Could you check a few things on this drawing? It's one solid part, dimensions in mm from its lowest x, y, z. A direction names the side the tool comes from. Give positions to 0.01 mm unless a question says otherwise; leave off trailing zeros. Loops run counter-clockwise (first coordinate to the right, second up) from the corner with the lowest first, then second, coordinate; pieces in that order, holes last.
Q1. I need wall thicknesses on probe 1 along Z at (x, y) = (25, 24); probe 2 along Z at (x, y) = (26.5, 2); probe 3 along Y at (x, z) = (19, 37.5). Which ranges of each line are inside material? Lowest first, please.
Q2. I'm going to push flat-ended pins straight in: P1, Ø6, axis at x = 31.5, y = 6.5, coming from the -Z side; P2, Ø1.3, axis at y = 17.5, z = 48.5, coming from the +X side; P3, Ø5, axis at x = 7, z = 20.5, coming from the +Y side; P4, Ø1.5, axis at x = 19.5, z = 24.5, coming from the +Y side. Where does each tip first touch, or does it pass through?
Q3. Suppose I cut it at B-B (x = 18.5). List the corners of the cut face in (y, z) for me, and give its area (3 significant figures).
Q4. Suppose I cut it at D-D (y = 23). List the corners of the cut face in (x, z) for me, and give its area (3 significant figures).
Q5. Suppose I cut it at A-A (y = 18.5). List the corners of the cut face in (x, z) for me.
Q6. For the marked faces 1 and 2, which set-ups out of +Z, -Z, +X, -X, +Y, -Y let a thin tool reach every point of the face, with its end or its side?
Q7. Suppose I cut it at C-C (z = 36). List the corners of the cut face in (x, y) for me, and give its area (3 significant figures).
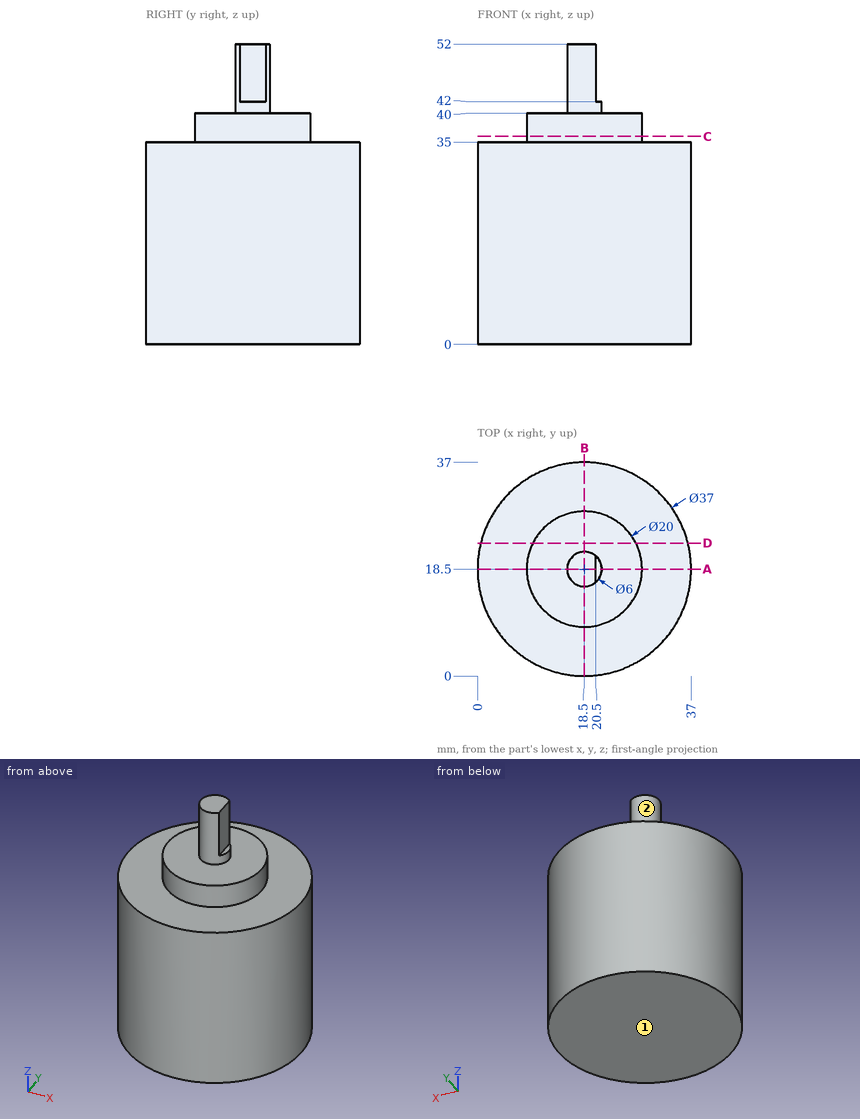
Solutions:
1. probe 1: z = 0 to 40
1. probe 2: z = 0 to 35
1. probe 3: y = 8.51 to 28.49
2. P1: stops at z = 0
2. P2: stops at x = 20.5
2. P3: stops at y = 34.66
2. P4: stops at y = 37
3. outline: (0, 0) - (37, 0) - (37, 35) - (28.5, 35) - (28.5, 40) - (21.5, 40) - (21.5, 52) - (15.5, 52) - (15.5, 40) - (8.5, 40) - (8.5, 35) - (0, 35) - close
3. area: 1,470 mm2
4. outline: (0.56, 0) - (36.44, 0) - (36.44, 35) - (27.43, 35) - (27.43, 40) - (9.57, 40) - (9.57, 35) - (0.56, 35) - close
4. area: 1,350 mm2
5. outline: (0, 0) - (37, 0) - (37, 35) - (28.5, 35) - (28.5, 40) - (21.5, 40) - (21.5, 42) - (20.5, 42) - (20.5, 52) - (15.5, 52) - (15.5, 40) - (8.5, 40) - (8.5, 35) - (0, 35) - close
6. face 1: -Z, +X, -X, +Y, -Y
6. face 2: +Z
7. outline: circle Ø20 at (18.5, 18.5)
7. area: 314 mm2
